Solid Edge part; units mm, degrees
sketch "Sketch1" plane through (0, 0, 0) normal (0, -1, 0) x (1, 0, 0)
  line L0 (15, -15) -> (15, 15)
  line L1 (15, 15) -> (-15, 15)
  line L2 (-15, 15) -> (-15, -15)
  line L3 (-15, -15) -> (15, -15)
extrude "Protrusion1" add sketch "Sketch1" against normal blind 30
sketch "Sketch2" plane through (0, 0, 0) normal (0, -1, 0) x (1, 0, 0)
  line L0 (10, 10) -> (-10, 10)
  line L1 (-10, 10) -> (-10, -10)
  line L2 (-10, -10) -> (10, -10)
  line L3 (10, -10) -> (10, 10)
extrude "ExtrudedCutout_1" cut sketch "Sketch2" against normal blind 30
sketch "Sketch3" plane through (0, 10, 0) normal (0, -1, 0) x (1, 0, 0)
  line L0 (18, 12) -> (40, 12)
  line L1 (40, -12) -> (18, -12)
  line L2 (15, -15) -> (15, 15)
  arc A0 (40, 12) -> (40, -12) centre (40, 0) cw
  arc A1 (15, -15) -> (18, -12) centre (18, -15) cw
  arc A2 (18, 12) -> (15, 15) centre (18, 15) cw
extrude "ExtrudedProtrusion_2" add sketch "Sketch3" against normal blind 10
sketch "Sketch4" plane through (0, 10, 0) normal (0, -1, 0) x (1, 0, 0)
  circle A0 centre (40, 0) radius 5
extrude "ExtrudedCutout_2" cut sketch "Sketch4" against normal blind 10
sketch "Sketch5" plane through (33.5, 10, 0) normal (0, -1, 0) x (1, 0, 0)
  line L0 (-51.5, 12) -> (-73.5, 12)
  line L1 (-73.5, -12) -> (-51.5, -12)
  line L2 (-48.5, -15) -> (-48.5, 15)
  arc A0 (-73.5, -12) -> (-73.5, 12) centre (-73.5, 0) cw
  arc A1 (-51.5, -12) -> (-48.5, -15) centre (-51.5, -15) cw
  arc A2 (-48.5, 15) -> (-51.5, 12) centre (-51.5, 15) cw
extrude "ExtrudedProtrusion_3" add sketch "Sketch5" against normal blind 10
sketch "Sketch6" plane through (33.5, 10, 0) normal (0, -1, 0) x (1, 0, 0)
  circle A0 centre (-73.5, 0) radius 5
extrude "ExtrudedCutout_3" cut sketch "Sketch6" against normal blind 10
sketch "Sketch7" plane through (0, 30, 0) normal (0, 1, 0) x (-1, 0, 0)
  line L0 (-24.5, -70) -> (-15, -15)
  line L1 (-15, -15) -> (15, -15)
  line L2 (24.5, -70) -> (15, -15)
  line L3 (15, -70) -> (24.5, -70)
  line L4 (15, -70) -> (-15, -70)
  line L5 (-15, -70) -> (-24.5, -70)
extrude "ExtrudedProtrusion_4" add sketch "Sketch7" against normal blind 22.5
sketch "Sketch8" plane through (-7.5, 5, 0) normal (-1, 0, 0) x (0, -1, 0)
  line L0 (20, -70) -> (5, -15)
  line L1 (-2.5, -15) -> (5, -15)
  line L2 (-2.5, -15) -> (-2.5, -70)
  line L3 (-2.5, -70) -> (20, -70)
extrude "ExtrudedProtrusion_7" add sketch "Sketch8" against normal blind 15
Geometry check sheet. Reference: the model listing, model coordinates, mm. A direction names the side the tool comes from. Round coordinates to 2 decimals unless told otherwise and drop trailing zeros. Order: outer loops, then holes, each group sorted by start corner. A loop starts at its lowest first (then second) coordinate and runs counter-clockwise, first axis right, second up. Notation, with made-up numbers: (-5, 74.25) - (27, 74.25) arc R20 cw to (27, 94.25) - close; hole circle Ø6 at (29, 77.25). An arc over 180 degrees is marked (long way). Use a Markdown table: item, result. Add a question column.
(1) Material ranges on line 1 along Z through (x, y) = (40, 14); line 2 along Y through (x, z) = (11, -38.5); line 3 along X through (y, z) = (13.5, -6), recorded low to high. Write a range as [from, to].
(2) Sectioned sample at B-B, the plane x = -5.5. Enter the section's corners in (y, z), and give its area (3 significant figures).
(3) Sectioned sample at C-C, the plane y = 16. Enter the section's corners in (x, z), and give its area (3 significant figures).
(4) Sectioned sample at A-A, the plane z = 0. Enter the section's corners in (x, y).
(5) Release check for a two-part mould opening along Z. For faces 4 (the flat face through (0.2, 0, 10.2)), 5 (the flat face through (0, 13, -70)), 6 (the flat face through (10, 15, 0)) record: pulls with the +Z half, pulls with the -Z half, needs draft (parallel to the pull), parting line crosses it, or undercut.
(6) Sectioned sample at D-D, the plane z = -52.5. Enter the section's corners in (x, y).
(7) Depth check by flat-ended pin: pin 1 (8 mm diameter, centred on y = 27, z = -3.5, fed in from +X); pin 2 (3 mm diameter, centred on y = 2.5, z = 5.5, fed in from -X); pin 3 (11.5 mm diameter, centred on x = 40, z = 0, fed in from +Y). Enter the tip coordinate at first touch or a pass-through.
(8) Tool access check on faces 1 (the flat face through (-29, 15, 12)), 2 (the flat face through (7.5, -1, -48)), 3 (the cylindrical face through (-15.86, 14.93, -12.9)). Record the directions out of +Z, -Z, +X, -X, +Y, -Y that give a thin tool (end or side, any length) a straight path to the whole face; none if there is none.
Answers below:
| question | item | result |
|---|---|---|
| 1 | line 1 | [-12, -5], [5, 12] |
| 1 | line 2 | [7.5, 30] |
| 1 | line 3 | [-50.39, -10], [10, 50.39] |
| 2 | outline | (-15, -70) - (30, -70) - (30, -10) - (0, -10) - (0, -15) - close; (0, 10) - (30, 10) - (30, 15) - (0, 15) - close |
| 2 | area | 2,360 mm² |
| 3 | outline | (-40, -12) - (-18, -12) arc R3 cw to (-15, -15) - (-24.5, -70) - (24.5, -70) - (15, -15) arc R3 cw to (18, -12) - (40, -12) arc R12 ccw to (40, 12) - (18, 12) arc R3 cw to (15, 15) - (-15, 15) arc R3 cw to (-18, 12) - (-40, 12) arc R12 ccw to start; hole circle Ø10 at (-40, 0); hole (-10, -10) - (10, -10) - (10, 10) - (-10, 10) - close; hole circle Ø10 at (40, 0) |
| 3 | area | 4,180 mm² |
| 4 | outline | (-52, 10) - (-45, 10) - (-45, 20) - (-52, 20) - close; (-35, 10) - (-15, 10) - (-15, 0) - (-10, 0) - (-10, 30) - (-15, 30) - (-15, 20) - (-35, 20) - close; (10, 0) - (15, 0) - (15, 10) - (35, 10) - (35, 20) - (15, 20) - (15, 30) - (10, 30) - close; (45, 10) - (52, 10) - (52, 20) - (45, 20) - close |
| 5 | face 4 | needs draft |
| 5 | face 5 | pulls with the -Z half |
| 5 | face 6 | undercut |
| 6 | outline | (-21.48, 7.5) - (-7.5, 7.5) - (-7.5, -10.23) - (7.5, -10.23) - (7.5, 7.5) - (21.48, 7.5) - (21.48, 30) - (-21.48, 30) - close |
| 7 | pin 1 | x = 15 |
| 7 | pin 2 | x = -15 |
| 7 | pin 3 | y = 20 |
| 8 | face 1 | +Z, -X, +Y, -Y |
| 8 | face 2 | -Z, +X, -Y |
| 8 | face 3 | -X, +Y, -Y |
